```python
from build123d import *

# Parameters (mm, degrees)
SKETCH2_R               = 15
SKETCH2_R_2             = 13.5
BOSS_EXTRUDE2_DEPTH     = 75
CUT_EXTRUDE1_DEPTH      = 78.942286341
CUT_EXTRUDE1_DEPTH_BACK = 78.942286341
SKETCH4_RX              = 3.5
SKETCH4_RY              = 2.5
CUT_EXTRUDE2_DEPTH      = 78.942286475
CUT_EXTRUDE2_DEPTH_BACK = 78.942286475
SKETCH5_RX              = 3.5
SKETCH5_RY              = 2.5
CUT_EXTRUDE3_DEPTH      = 78.942286475
CUT_EXTRUDE3_DEPTH_BACK = 78.942286475
SKETCH6_W               = 25
SKETCH6_H               = 15


with BuildPart() as part:
    # Sketch2 → Boss-Extrude2 (new body)
    with BuildSketch(Plane(origin=(0, 0, 0), x_dir=(1, 0, 0), z_dir=(0, 1, 0))):
        with Locations(Location((0, 0, 0), (0, 0, 270))):
            Circle(SKETCH2_R)
        with Locations(Location((0, 0, 0), (0, 0, 270))):
            Circle(SKETCH2_R_2, mode=Mode.SUBTRACT)
    extrude(amount=BOSS_EXTRUDE2_DEPTH)

    # Sketch4 → Cut-Extrude1 (cut, two sides: drawn at the far end of the back side and taken through both)
    with BuildSketch(Plane.XY.offset(-CUT_EXTRUDE1_DEPTH_BACK)):
        with Locations((0, 10)):
            Ellipse(SKETCH4_RX, SKETCH4_RY)
    extrude(amount=CUT_EXTRUDE1_DEPTH + CUT_EXTRUDE1_DEPTH_BACK, mode=Mode.SUBTRACT)

    # Sketch5 → Cut-Extrude2 (cut, two sides: drawn at the far end of the back side and taken through both)
    with BuildSketch(Plane(origin=(0, 0, 0), x_dir=(0, 0, -1), z_dir=(1, 0, 0)).offset(-CUT_EXTRUDE2_DEPTH_BACK)):
        with Locations(Location((0, 10), (0, 0, 180))):
            Ellipse(SKETCH5_RX, SKETCH5_RY)
    extrude(amount=CUT_EXTRUDE2_DEPTH + CUT_EXTRUDE2_DEPTH_BACK, mode=Mode.SUBTRACT)

    # Sketch6 → Cut-Extrude3 (cut, two sides: drawn at the far end of the back side and taken through both)
    with BuildSketch(Plane.XY.offset(-CUT_EXTRUDE3_DEPTH_BACK)):
        with Locations((0, 67.5)):
            Rectangle(SKETCH6_W, SKETCH6_H)
    extrude(amount=CUT_EXTRUDE3_DEPTH + CUT_EXTRUDE3_DEPTH_BACK, mode=Mode.SUBTRACT)


solid = part.part
```
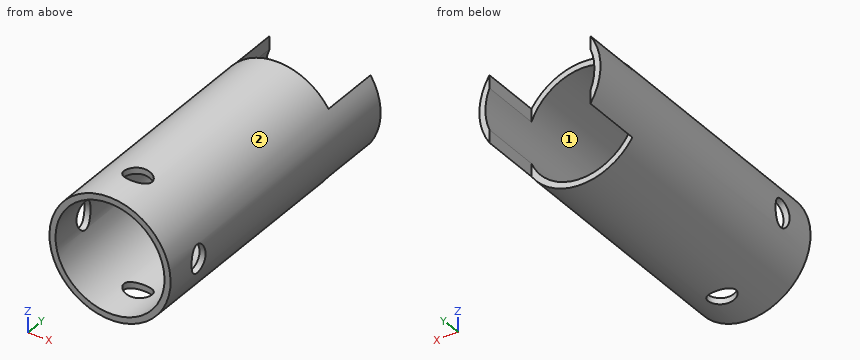
Design review of the part built by this model. Coordinates are the model's own, in mm. Face numbers are marked on the shaded views. Give positions to 0.01 mm unless a question says otherwise; leave off trailing zeros. Order: outer loops, then holes, each group sorted by start corner. A loop starts at its lowest first (then second) coordinate and runs counter-clockwise, first axis right, second up. Notation, with made-up numbers: (1.25, -16) -> (10.25, -16) arc R30 cw to (10.25, 21) -> close; hole circle Ø6 at (10.5, 40.25). An arc over 180 degrees is marked (long way). Write each question's results on one line, items separated by ' | '. Start each with the question number.
Q1. Wall thickness on L1, parallel to X at y = 44, z = 0; L2, parallel to Z at x = -6, y = 28.5: over which ranges is each line inside the solid? List them lowest first. Write a range as from..to.
Q2. Add section A-A on y = 65. Give the boundary of the cut face in (x, z), and give its area (3 significant figures).
Q3. For pin 1 (2 mm diameter, centred on y = 47.5, z = -10.5, fed in from -X); pin 2 (12 mm diameter, centred on y = 63, z = 9, fed in from +X); pin 3 (3.5 mm diameter, centred on y = 68.5, z = 7, fed in from -X), all flat-tipped, find the tip position at first contact; note any pin that passes through.
Q4. Add section C-C on z = -7. Give the boundary of the cut face in (x, y), and give its area (3 significant figures).
Q5. Add section D-D on z = 0. State how many separate pieces and enclosed holes the cut face has, and give its area (3 significant figures).
Q6. Add section B-B on x = -8. Give the boundary of the cut face in (y, z), and give its area (3 significant figures).
Q7. Mouldability with a two-part tool opening along Z and no side actions: class the marked faces 1 and 2 as +Z half, -Z half, draft (parallel to the pull), parting line (faces both ways), or undercut.
Found:
1) L1: x = -15..-13.5, 13.5..15 | L2: z = -13.75..-12.09, 12.09..13.75
2) outline: (-12.5, -8.29) -> (-12.5, -5.1) arc R13.5 cw to (-12.5, 5.1) -> (-12.5, 8.29) arc R15 ccw to start; (12.5, -8.29) arc R15 ccw to (12.5, 8.29) -> (12.5, 5.1) arc R13.5 cw to (12.5, -5.1) -> close | area: 42.6 mm2
3) pin 1: stops at x = -11.61 | pin 2: stops at x = 14.7 | pin 3: stops at x = -14.05
4) outline: (-13.27, 0) -> (-11.54, 0) -> (-11.54, 60) -> (-12.5, 60) -> (-12.5, 75) -> (-13.27, 75) -> close; (11.54, 0) -> (13.27, 0) -> (13.27, 75) -> (12.5, 75) -> (12.5, 60) -> (11.54, 60) -> close | area: 230 mm2
5) separate pieces: 4 | enclosed holes: 0 | area: 210 mm2
6) outline: (0, -12.69) -> (60, -12.69) -> (60, -10.87) -> (0, -10.87) -> close; (0, 10.87) -> (60, 10.87) -> (60, 12.69) -> (0, 12.69) -> close | area: 218 mm2
7) face 1: undercut | face 2: parting line
